The model under review builds one solid part; all positions refer to its coordinate system, in mm. Face numbers are marked on the shaded views. A direction names the side the tool comes from. Coordinates: 2 decimals unless noted, no trailing zeros. Loops run counter-clockwise (first coordinate to the right, second up) from the corner with the lowest first, then second, coordinate; pieces in that order, holes last. Notation, with made-up numbers: (43.5, 79) - (72.5, 79) arc R5 ccw to (72.5, 83) - close; hole circle Ø1 at (57, -27.5). An arc over 180 degrees is marked (long way). One line per item, written item: value. Start each with the question number.
1. For the marked faces 1, 2, 3 and 4, list the 3-axis set-ups (+Z, -Z, +X, -X, +Y, -Y) from which the entire face can be reached by the end or side of a thin tool; tool diameter is ignored.
2. We need section A-A, the plane y = 24.5. Give the boundary of the cut face in (x, z).
3. Mouldability with a two-part tool opening along Y and no side actions: class the marked faces 5, 6 and 7 as +Y half, -Y half, draft (parallel to the pull), parting line (faces both ways), or undercut.
4. To check wall thickness, follow line 1 (Y direction, x = 43, z = 54); line 2 (Y direction, x = -52, z = 16); line 3 (Z direction, x = 0, y = 2). State the ranges of each line that lie inside material, in increasing order.
5. We need section B-B, the plane y = 80.5. Give the boundary of the cut face in (x, z), then the cut area to 3 significant figures.
6. We need section C-C, the plane y = 151. Give the boundary of the cut face in (x, z), then the cut area to 3 significant figures.
7. Insertion check: P1, Ø17.5, axis at x = -2.5, z = -3, coming from the -Y side; P2, Ø10, axis at x = -33, y = 90, coming from the +Z side; P3, Ø18.5, axis at y = 4.5, z = -15.5, coming from the +X side. Each pin has a flat end and moves straight along its axis. Give the tip position at first contact, or say it passes through.
Autodesk Inventor part; units mm, degrees
ref_plane "YZ Plane" through (0, 0, 0) normal (1, 0, 0) x (0, 1, 0)
ref_plane "XZ Plane" through (0, 0, 0) normal (0, 1, 0) x (-1, 0, 0)
ref_plane "XY Plane" through (0, 0, 0) normal (0, 0, 1) x (1, 0, 0)
sketch "Sketch1" plane through (0, 0, 0) normal (0, 1, 0) x (-1, 0, 0)
  line L0 (-61, 66) -> (61, 66)
  line L1 (66, 61) -> (66, -61)
  line L2 (61, -66) -> (-61, -66)
  line L3 (-66, -61) -> (-66, 61)
  line L4 (-66, 66) -> (66, -66) construction
  line L5 (66, 66) -> (-66, -66) construction
  circle A0 centre (0, 0) radius 72.5 construction
  circle A1 centre (51.2652, 51.2652) radius 4
  circle A2 centre (51.2652, -51.2652) radius 4
  line L6 (0, 66) -> (0, 0) construction
  circle A3 centre (-51.2652, 51.2652) radius 4
  circle A4 centre (-51.2652, -51.2652) radius 4
  arc A5 (61, -66) -> (66, -61) centre (61, -61) ccw
  arc A6 (-66, -61) -> (-61, -66) centre (-61, -61) ccw
  line L7 (0, 0) -> (66, 0) construction
  arc A7 (66, 61) -> (61, 66) centre (61, 61) ccw
  arc A8 (-61, 66) -> (-66, 61) centre (-61, 61) ccw
  dimension "d0" = 132
  dimension "d1" = 132
  dimension "d3" = 8
  dimension "d4" = 8
  dimension "d5" = 5
  dimension "d47" = 145
extrude "Extrusion1" add sketch "Sketch1" along normal blind 17
sketch "Sketch2" plane through (0, 17, 0) normal (0, 1, 0) x (1, 0, 0)
  circle A0 centre (0, 0) radius 65
  dimension "d8" = 130
extrude "Extrusion2" add sketch "Sketch2" along normal blind 99
sketch "Sketch3" plane through (0, 116, 0) normal (0, 1, 0) x (1, 0, 0)
  line L0 (62, 67) -> (-62, 67)
  line L1 (-67, 62) -> (-67, -62)
  line L2 (-62, -67) -> (62, -67)
  line L3 (67, -62) -> (67, 62)
  line L4 (-67, 67) -> (67, -67) construction
  arc A0 (-67, -62) -> (-62, -67) centre (-62, -62) ccw
  arc A1 (-62, 67) -> (-67, 62) centre (-62, 62) ccw
  arc A2 (67, 62) -> (62, 67) centre (62, 62) ccw
  arc A3 (62, -67) -> (67, -62) centre (62, -62) ccw
  line L5 (51, -51) -> (-51, -51) construction
  line L6 (-51, -51) -> (-51, 51) construction
  line L7 (-51, 51) -> (51, 51) construction
  line L8 (51, 51) -> (51, -51) construction
  line L9 (51, -51) -> (-51, 51) construction
  line L10 (-51, -51) -> (51, 51) construction
  line L11 (57, -57) -> (-57, -57) construction
  line L12 (-57, -57) -> (-57, 57) construction
  line L13 (-57, 57) -> (57, 57) construction
  line L14 (57, 57) -> (57, -57) construction
  line L15 (-57, -57) -> (-51, -51) construction
  line L16 (0, 0) -> (0, 51) construction
  line L17 (0, 0) -> (51, 0) construction
  line L18 (-54, -54) -> (-47.1057, -47.1057) construction
  line L19 (-51, -51) -> (-57, -57) construction
  line L20 (-54.8943, -47.1057) -> (-60.8943, -53.1057)
  line L21 (-53.1057, -60.8943) -> (-47.1057, -54.8943)
  arc A4 (-47.1057, -54.8943) -> (-54.8943, -47.1057) centre (-51, -51) ccw
  arc A5 (-60.8943, -53.1057) -> (-53.1057, -60.8943) centre (-57, -57) ccw
  line L22 (51, -51) -> (54, -54) construction
  line L23 (54, -54) -> (47.1057, -47.1057) construction
  line L24 (51, -51) -> (57, -57) construction
  line L25 (47.1057, -54.8943) -> (53.1057, -60.8943)
  line L26 (60.8943, -53.1057) -> (54.8943, -47.1057)
  arc A6 (54.8943, -47.1057) -> (47.1057, -54.8943) centre (51, -51) ccw
  arc A7 (53.1057, -60.8943) -> (60.8943, -53.1057) centre (57, -57) ccw
  line L27 (51, 51) -> (54, 54) construction
  line L28 (54, 54) -> (47.1057, 47.1057) construction
  line L29 (51, 51) -> (57, 57) construction
  line L30 (54.8943, 47.1057) -> (60.8943, 53.1057)
  line L31 (53.1057, 60.8943) -> (47.1057, 54.8943)
  arc A8 (47.1057, 54.8943) -> (54.8943, 47.1057) centre (51, 51) ccw
  arc A9 (60.8943, 53.1057) -> (53.1057, 60.8943) centre (57, 57) ccw
  line L32 (-51, 51) -> (-57, 57) construction
  line L33 (-51, 51) -> (-54, 54) construction
  line L34 (-54, 54) -> (-47.1057, 47.1057) construction
  line L35 (-51, 51) -> (-57, 57) construction
  line L36 (-47.1057, 54.8943) -> (-53.1057, 60.8943)
  line L37 (-60.8943, 53.1057) -> (-54.8943, 47.1057)
  arc A10 (-54.8943, 47.1057) -> (-47.1057, 54.8943) centre (-51, 51) ccw
  arc A11 (-53.1057, 60.8943) -> (-60.8943, 53.1057) centre (-57, 57) ccw
  point P0 (-67, 0)
  point P1 (0, 67)
  point P2 (-60.8943, -60.8943)
  dimension "d22" = 5
  dimension "d48" = 102
  dimension "d49" = 102
  dimension "d50" = 114
  dimension "d51" = 114
  dimension "d53" = 9.75
  dimension "d76" = 9.75
  dimension "d77" = 9.75
  dimension "d78" = 9.75
  dimension "d79" = 11.0147
  dimension "d80" = 19.5
extrude "Extrusion3" add sketch "Sketch3" along normal blind 15
sketch "Sketch4" plane through (0, 131, 0) normal (0, 1, 0) x (1, 0, 0)
  circle A0 centre (0, 0) radius 55
  dimension "d19" = 110
extrude "Extrusion4" add sketch "Sketch4" along normal blind 5
sketch "Sketch5" plane through (0, 136, 0) normal (0, 1, 0) x (1, 0, 0)
  arc A0 (-3, 10.583) -> (3, 10.583) centre (0, 0) ccw
  line L0 (0, -11) -> (0, 13.5) construction
  line L1 (-3, 8.5) -> (3, 8.5)
  line L2 (3, 8.5) -> (3, 10.583)
  line L3 (-3, 10.583) -> (-3, 8.5)
  line L4 (-3, 8.5) -> (3, 13.5) construction
  line L5 (3, 8.5) -> (-3, 13.5) construction
  dimension "d54" = 22
extrude "Extrusion5" add sketch "Sketch5" along normal blind 52
sketch "Sketch7" plane through (0, 0, 0) normal (0, 0, 1) x (1, 0, 0)
  line L0 (-65, 106) -> (-65, 103.5)
  line L1 (-65, 106) -> (-64.5, 106)
  line L2 (-64.5, 106) -> (-64.5, 103.5)
  line L3 (-64.5, 103.5) -> (-65, 103.5)
  line L4 (-65, 17) -> (-65, 37) construction
  line L5 (-65, 37) -> (-64.5, 37)
  line L6 (-64.5, 37) -> (-64.5, 39.5)
  line L7 (-64.5, 39.5) -> (-65, 39.5)
  line L8 (-65, 39.5) -> (-65, 37)
  line L9 (0, -27.2) -> (0, 163.2)
  line L10 (-65, 121) -> (-65, 106) construction
  point P0 (0, 0)
  dimension "d35" = 2.5
  dimension "d36" = 0.5
  dimension "d37" = 20
  dimension "d38" = 0.5
  dimension "d39" = 2.5
  dimension "d41" = 15
revolve "Revolution1" cut sketch "Sketch7" angle 360 about axis through (0, -10, 0) along (0, 1, 0)
sketch "Sketch8" plane through (0, 0, 0) normal (0, -1, 0) x (1, 0, 0)
  arc A0 (-3, 10.583) -> (3, 10.583) centre (0, 0) ccw
  line L0 (0, -11) -> (0, 13.7) construction
  line L1 (3, 10.583) -> (3, 13.7)
  line L2 (3, 13.7) -> (-3, 13.7)
  line L3 (-3, 13.7) -> (-3, 10.583)
  line L4 (-3, 8.3) -> (3, 13.7) construction
  line L5 (3, 8.3) -> (-3, 13.7) construction
  dimension "d72" = 22
  dimension "d73" = 24.7
  dimension "d74" = 6
extrude "Extrusion7" cut sketch "Sketch8" against normal blind 62
sketch "Sketch11" plane through (0, 136, 0) normal (0, 1, 0) x (1, 0, 0)
  circle A0 centre (0, 0) radius 12
  dimension "d60" = 24
extrude "Extrusion9" add sketch "Sketch11" along normal blind 2
chamfer "Chamfer1" distance 1 angle 45 1 edges at (0, 188, 11)
sketch "Sketch12" plane through (0, 136, 0) normal (0, 1, 0) x (1, 0, 0)
  circle A0 centre (0, 0) radius 35
  circle A1 centre (0, 0) radius 40
  dimension "d66" = 70
extrude "Extrusion10" cut sketch "Sketch12" against normal blind 0.0001
sketch "Sketch13" plane through (0, 0, 0) normal (0, -1, 0) x (1, 0, 0)
  circle A0 centre (0, 0) radius 55
  dimension "d69" = 110
extrude "Extrusion11" cut sketch "Sketch13" against normal blind 6
properties part number "PX130-GEARBOX"
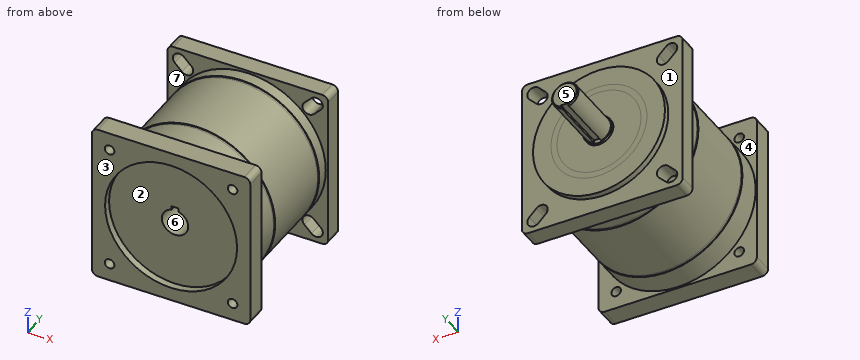
Findings below:
1. face 1: +Y
1. face 2: -Y
1. face 3: +Z, -Z, +X, -X, -Y
1. face 4: none
2. outline: circle Ø130 at (0, 0); hole (-3, 10.58) arc R11 ccw (long way) to (3, 10.58) - (3, 13.7) - (-3, 13.7) - close
3. face 5: +Y half
3. face 6: draft
3. face 7: undercut
4. line 1: 0 to 17, 116 to 131
4. line 2: 6 to 136
4. line 3: -66 to -55, 55 to 66
5. outline: circle Ø130 at (0, 0)
5. area: 13,300 mm2
6. outline: (-3, -10.58) - (-3, -8.5) - (3, -8.5) - (3, -10.58) arc R11 ccw (long way) to start
6. area: 366 mm2
7. P1: y = 6
7. P2: z = 58.66
7. P3: x = 66
